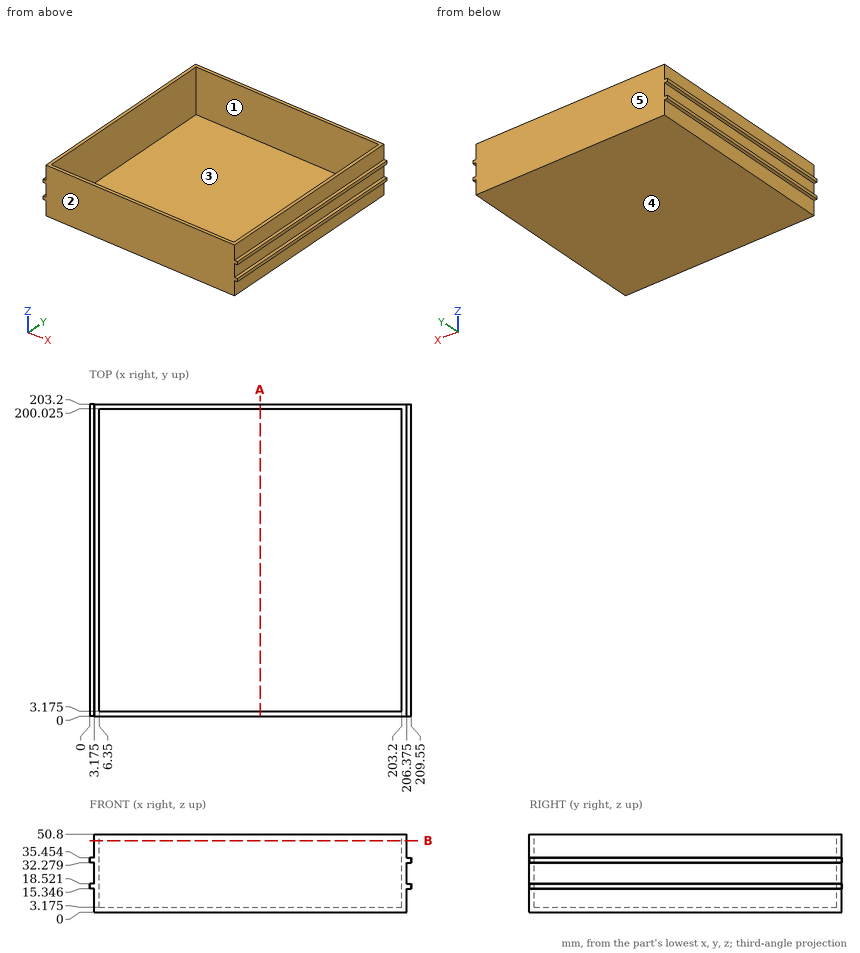
Here's the drawing with two shaded views (mm, measured from the low corner). I have some questions. A direction names the side the tool comes from. Coordinates: 2 decimals unless noted, no trailing zeros. Loops run counter-clockwise (first coordinate to the right, second up) from the corner with the lowest first, then second, coordinate; pieces in that order, holes last. Notation, with made-up numbers: (-24, -32.5) -> (30, -32.5) arc R13 ccw to (30, -23.5) -> close; hole circle Ø4 at (55, 52). An arc over 180 degrees is marked (long way). Answer as a JSON object with one key per item and string values.
1) For the marked faces 1 and 2, which set-ups out of +Z, -Z, +X, -X, +Y, -Y let a thin tool reach every point of the face, with its end or its side?
Results:
{"face 1": "+Z", "face 2": "+Z, -Z, +X, -X, -Y"}
2) If I drill on line 1 (X direction, y = 106.5, z = 41.5) (3 decimals); line 2 (Y direction, x = 68, z = 14) (3 decimals); line 3 (X direction, y = 42, z = 33), over which ranges is the centre line in solid material (lowest first)?
Results:
{"line 1": "x = 3.175 to 6.35, 203.2 to 206.375", "line 2": "y = 0 to 3.175, 200.025 to 203.2", "line 3": "x = 0 to 6.35, 203.2 to 209.55"}
3) Imagine slicing it at B-B (z = 46.5). Please give me the cut outline in (x, y) (3 decimals), then the cut area to 3 significant figures.
Results:
{"outline": "(3.175, 0) -> (206.375, 0) -> (206.375, 203.2) -> (3.175, 203.2) -> close; hole (6.35, 3.175) -> (203.2, 3.175) -> (203.2, 200.025) -> (6.35, 200.025) -> close", "area": "2,540 mm^2"}
4) Imagine slicing it at A-A (x = 111). Please give me the cut outline in (y, z) (3 decimals).
Results:
{"outline": "(0, 0) -> (203.2, 0) -> (203.2, 50.8) -> (200.025, 50.8) -> (200.025, 3.175) -> (3.175, 3.175) -> (3.175, 50.8) -> (0, 50.8) -> close"}
5) Thinking about a two-plate mould opening in Y: for the marked faces 3, 4 and 5, which applies, pulls with the +Y half, pulls with the -Y half, needs draft (parallel to the pull), parting line crosses it, or undercut?
Results:
{"face 3": "undercut", "face 4": "needs draft", "face 5": "pulls with the +Y half"}
6) For P1, Ø10, axis at x = 27, z = 27.5, coming from the -Y side; P2, Ø1, axis at x = 2.5, y = 104.5, coming from the -Z side; P3, Ø1.5, axis at y = 76.5, z = 22.5, coming from the -X side (3 decimals); P4, Ø4.5, axis at y = 124.5, z = 40, coming from the +X side (3 decimals), each with a flat end and sliding along its axis, tell me the tip position at first contact or that it passes through.
Results:
{"P1": "stops at y = 0", "P2": "stops at z = 15.35", "P3": "stops at x = 3.175", "P4": "stops at x = 206.375"}
